Autodesk Inventor part; units mm, degrees
ref_plane "Work Plane1" through (2.75, 0, 0) normal (0, -1, 0) x (1, 0, 0)
ref_plane "YZ Plane" through (0, 0, 0) normal (1, 0, 0) x (0, 1, 0)
ref_plane "XZ Plane" through (0, 0, 0) normal (0, 1, 0) x (-1, 0, 0)
sketch "Skizze1" plane through (0, 0, 0) normal (0, 0, 1) x (1, 0, 0)
  line L0 (70, 12) -> (70, 0)
  line L1 (-40.5, 0) -> (70, 0)
  line L2 (-62.6, 0) -> (92.1, 0)
  line L3 (0, 14.4) -> (0, -2.4)
  line L4 (-40.5, 12) -> (-40.5, 0)
  line L5 (16, 12) -> (16, 0) construction
  line L6 (-62.6, 0) -> (92.1, 0)
  line L7 (-40.5, 12) -> (70, 12)
  dimension "d4" = 40.5
  dimension "d5" = 70
  dimension "d6" = 54
  dimension "d13" = 24
revolve "Körper" add sketch "Skizze1" angle 360 about axis through (-40.5, 0, 0) along (1, 0, 0)
thread "Gewinde1"
thread "Gewinde2"
chamfer "Fase1" distance 1.8414 distance2 3 1 edges at (70, -12, 0) measured on face at (70, 0.4821, 1.3341)
chamfer "Fase2" distance 1.8414 distance2 3 1 edges at (-40.5, -12, 0) measured on face at (31.1667, 11.9611, -0.9656)
ref_plane "Work Plane1" through (2.75, 0, 0) normal (0, -1, 0) x (1, 0, 0)
equation "\"d4\" = KOH"
equation "\"d5\" = NLG"
equation "\"d6\" = GEL"
equation "\"d13\" = GD"
equation "\"d1\" = KOH"
equation "\"d7\" = GEL + GAL"
equation "\"d10\" = -0.5 * SPD + 0.5 * GD"
equation "\"d12\" = -0.5 * SPD + 0.5 * GD"
equation "\"NLG\" = 70"
equation "\"GEL\" = 54"
equation "\"GAL\" = 0.61345 * PTC"
equation "\"SPD\" = 18"
equation "\"d0\" = GD"
equation "\"GUL\" = 0.61345 * PTC"
equation "\"KOH\" = 40.5"
equation "\"GD\" = 24"
equation "\"BDM\" = NND"
equation "\"GUL1\" = GUL"
equation "\"GAL1\" = GAL"
equation "\"d80\" = -GUL - GEL"
equation "\"d86\" = -KOH + GUL1"
equation "\"PTC\" = 3"
equation "\"THREADDIA\" = 24"
equation "\"TOA\" = 30deg"
equation "\"NND\" = 24"
equation "\"GD1\" = THREADDIA - 1.2269 * PTC"
properties part number "DIN 835 - M24 x 70" material "Stahl, weich"
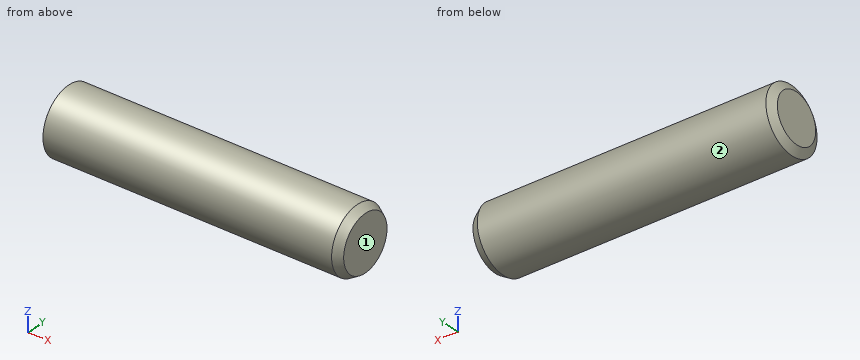
Build history of the part. All positions in model axes, mm. Face numbers are marked on the shaded views. Coordinates: 2 decimals unless noted, no trailing zeros. Order: outer loops, then holes, each group sorted by start corner. A loop starts at its lowest first (then second) coordinate and runs counter-clockwise, first axis right, second up. Notation, with made-up numbers: (-25.75, 68.25) -> (3.25, 68.25) arc R18 cw to (3.25, 79.25) -> close; hole circle Ø8 at (32, -40). An arc over 180 degrees is marked (long way). Answer in a Markdown table with one row per item. Add a question column.
Q1. Drop flat-ended pins along their axis: pin 1 (8 mm diameter, centred on x = 12, y = 9, fed in from -Z); pin 2 (1.5 mm diameter, centred on x = -24.5, z = -8, fed in from -Y); pin 3 (1 mm diameter, centred on x = 24, y = -5, fed in from +Z). Give the stop position or say it passes through.
Q2. Band-saw the part on A-A, the plane x = -6. List the corners of the cut face in (y, z), then the cut area to 3 significant figures.
Q3. Wall check: line 1 along Z through (x, y) = (-7.5, 0); line 2 along Y through (x, z) = (-23.5, -0.5); line 3 along Y through (x, z) = (44.5, -9.25). Give the ranges that are in metal, low to high. Write a range as [from, to].
Q4. Mould opens along Y. For the marked faces 1 and 2 say: +Y half, -Y half, draft (parallel to the pull), parting line (faces both ways), or undercut.
Answers follow:
| question | item | result |
|---|---|---|
| 1 | pin 1 | z = -10.91 |
| 1 | pin 2 | y = -9.56 |
| 1 | pin 3 | z = 11.12 |
| 2 | outline | circle Ø24 at (0, 0) |
| 2 | area | 452 mm^2 |
| 3 | line 1 | [-12, 12] |
| 3 | line 2 | [-11.99, 11.99] |
| 3 | line 3 | [-7.64, 7.64] |
| 4 | face 1 | draft |
| 4 | face 2 | parting line |
